The model under review builds one solid part; all positions refer to its coordinate system, in mm. A direction names the side the tool comes from. Round coordinates to 2 decimals unless told otherwise and drop trailing zeros. Write each loop counter-clockwise with the first axis right and the second up, starting at its lowest first coordinate (ties: lowest second). Pieces come first, ordered by that corner, then holes. Notation, with made-up numbers: M -8.75,-27.75 L 37.25,-27.75 A21 ccw 37.25,9.25 Z; hole C 76.5,27.25 d5. An arc over 180 degrees is marked long. Write item = value, one per line. Start each with the question number.
Item 1: Tool access review of faces 1 (the cylindrical face through (4.133, 1.301, 19.014)), 2 (the flat face through (-0.3, 5.1, 20)), 3 (the flat face through (0, 0, 14)): name each direction out of +Z, -Z, +X, -X, +Y, -Y from which nothing blocks a thin tool from reaching the whole face with its end or side.
Item 2: To check wall thickness, follow line 1 along Y through (x, z) = (0, 18.95); line 2 along X through (y, z) = (0, 13.5); line 3 along Z through (x, y) = (8.5, -3). State the ranges of each line that lie inside material, in increasing order.
Item 3: For pin 1 Ø4 at (y, z) = (-2.5, 3) entering from -X; pin 2 Ø7 at (x, y) = (0, 0) entering from -Z; pin 3 Ø5 at (x, z) = (15, 15) entering from +Y, all flat-tipped, find the tip position at first contact; note any pin that passes through.
Item 4: The part is to be moulded in two halves that separate along X. For faces 4 (the flat face through (8, 15, -6)), 5 (the cylindrical face through (4.368, 1.376, 19.014)), 6 (the cylindrical face through (-2.799, 21.317, 19.014)), say which applies: +X half, -X half, draft (parallel to the pull), parting line (faces both ways), or undercut.
Item 5: Take a section at C-C, the plane z = 7.5. Give the boundary of the cut face in (x, y).
Item 6: Take a section at D-D, the plane x = 9. Give the boundary of the cut face in (y, z), plus the area to 3 significant figures.
from build123d import *

# Parameters (mm, degrees)
F0_R      = 20.75
F1_DEPTH  = 20
F2_R      = 18
F3_DEPTH  = 6
F4_R      = 21.5
F5_DEPTH  = 2
F6_R      = 4.332633
F7_DEPTH  = 2
F8_R      = 16.5
F9_DEPTH  = 20
F10_R     = 4.852461
F10_R_2   = 4.579642
F11_DEPTH = 2
F12_R     = 4.001632
F13_DEPTH = 2


with BuildPart() as f1:
    # F0 (on Top) → F1 (new body)
    with BuildSketch(Plane.XY):
        Circle(F0_R)
    extrude(amount=F1_DEPTH)

    # F2 (on face) → F3 (join)
    with BuildSketch(Plane(origin=(0, 0, 0), x_dir=(1, 0, 0), z_dir=(0, 0, -1))):
        Circle(F2_R)
    extrude(amount=F3_DEPTH)

    # F4 (on face) → F5 (join)
    with BuildSketch(Plane.XY.offset(20)):
        Circle(F4_R)
    extrude(amount=-F5_DEPTH)

    # F6 (on face) → F7 (cut)
    with BuildSketch(Plane.XY.offset(20)):
        Circle(F6_R)
    extrude(amount=-F7_DEPTH, mode=Mode.SUBTRACT)

    # F8 (on face) → F9 (cut)
    with BuildSketch(Plane(origin=(0, 0, -6), x_dir=(1, 0, 0), z_dir=(0, 0, -1))):
        Circle(F8_R)
    extrude(amount=-F9_DEPTH, mode=Mode.SUBTRACT)

    # F10 (on face) → F11 (cut)
    with BuildSketch(Plane.XY.offset(20)):
        Circle(F10_R)
        Circle(F10_R_2, mode=Mode.SUBTRACT)
    extrude(amount=-F11_DEPTH, mode=Mode.SUBTRACT)

    # F12 (on face) → F13 (join)
    with BuildSketch(Plane.XY.offset(18)):
        Circle(F12_R)
    extrude(amount=F13_DEPTH)


solid = f1.part
Response values:
q1.face_1 = +Z
q1.face_2 = +Z, +X, -X, +Y, -Y
q1.face_3 = -Z
q2.line_1 = -21.5 to -4.85, -4.58 to -4.33, -4 to 4, 4.33 to 4.58, 4.85 to 21.5
q2.line_2 = -20.75 to -16.5, 16.5 to 20.75
q2.line_3 = 14 to 20
q3.pin_1 = -20.74
q3.pin_2 = 14
q3.pin_3 = 16.56
q4.face_4 = draft
q4.face_5 = undercut
q4.face_6 = parting line
q5.outline = C 0,0 d41.5; hole C 0,0 d33
q6.outline = M -19.53,18 L -18.7,18 L -18.7,0 L -15.59,0 L -15.59,-6 L -13.83,-6 L -13.83,14 L 13.83,14 L 13.83,-6 L 15.59,-6 L 15.59,0 L 18.7,0 L 18.7,18 L 19.53,18 L 19.53,20 L -19.53,20 Z
q6.area = 385 mm2
